Read the model definition and answer for the solid it produces. Units are mm, in the model's axes. A direction names the side the tool comes from. Give positions to 0.01 mm unless a question says otherwise; leave off trailing zeros. Loops run counter-clockwise (first coordinate to the right, second up) from the corner with the lowest first, then second, coordinate; pieces in that order, holes last. Notation, with made-up numbers: (1, -19) - (7, -19) arc R31 cw to (7, 9) - close; hole circle Ø8 at (2.25, 47.25). An arc over 180 degrees is marked (long way). Use a Markdown table: item, result. Add a question column.
Item 1: Consider probe 1 along X at (y, z) = (2.3, 75); probe 2 along Z at (x, y) = (-39, 2.5); probe 3 along X at (y, z) = (-2.5, 42). Determine where each line is inside the solid, lowest interval first. Write a range as [from, to].
Item 2: For a pull along X with two mould halves and no side action, classify faces 1 (the face through (45, 0, 120)), 2 (the face through (50, 0, 59)), 3 (the face through (-1, 0, 70)) as +X half, -X half, draft (parallel to the pull), parting line (faces both ways), or undercut.
Item 3: A cutting plane is placed at C-C (y = -0.85). Determine the outline of the cut face in (x, z), plus the area to 3 significant figures.
Item 4: Which of the six approach directions +Z, -Z, +X, -X, +Y, -Y give full straight-line access (tool end or side, diameter ignored) to faces 4 (the face through (-1, 0, 0)), 5 (the face through (-40, 0, 100)), 6 (the face through (-45, 0, 120)), 7 (the face through (40, 0, 40)), 8 (the face through (45, 1, 75))?
Item 5: Each of these flat-tipped pins is pushed along its axis until it touches: P1, Ø1.8, axis at x = -1.5, y = -1.5, coming from the +Z side; P2, Ø4, axis at x = 44.5, z = 75, coming from the +Y side. Where does it stop, or does it pass through?
Item 6: A cutting plane is placed at B-B (z = 62.5). Determine the outline of the cut face in (x, y), plus the area to 3 significant figures.
Item 7: A cutting plane is placed at A-A (x = -24). Determine the outline of the cut face in (y, z), plus the area to 3 significant figures.
Item 8: A cutting plane is placed at D-D (x = -45). Determine the outline of the cut face in (y, z).
from build123d import *

# Parameters (mm, degrees)
SKETCH1_W           = 80
SKETCH1_H           = 60
BOSS_EXTRUDE1_DEPTH = 3
SKETCH2_R           = 4
CUT_EXTRUDE1_DEPTH  = 2


with BuildPart() as part:
    # Sketch1 → Boss-Extrude1 (new, symmetric)
    with BuildSketch(Plane(origin=(0, 0, 0), x_dir=(1, 0, 0), z_dir=(0, 1, 0))):
        Polygon((-50, 0), (50, 0), (50, -120), (40, -120), (40, -80), (-40, -80), (-40, -120), (-50, -120), align=None)
        with Locations((0, -40)):
            Rectangle(SKETCH1_W, SKETCH1_H, mode=Mode.SUBTRACT)
    extrude(amount=BOSS_EXTRUDE1_DEPTH, both=True)

    # Sketch2 → Cut-Extrude1 (cut)
    with BuildSketch(Plane(origin=(0, 3, 0), x_dir=(1, 0, 0), z_dir=(0, 1, 0))):
        with Locations(Location((-45, -75, 0), (0, 0, 270))):
            Circle(SKETCH2_R)
        with Locations(Location((45, -75, 0), (0, 0, 270))):
            Circle(SKETCH2_R)
    extrude(amount=-CUT_EXTRUDE1_DEPTH, mode=Mode.SUBTRACT)


solid = part.part
Geometry says:
| question | item | result |
|---|---|---|
| 1 | probe 1 | [-50, -49], [-41, 41], [49, 50] |
| 1 | probe 2 | [0, 10], [70, 80] |
| 1 | probe 3 | [-50, -40], [40, 50] |
| 2 | face 1 | draft |
| 2 | face 2 | +X half |
| 2 | face 3 | undercut |
| 3 | outline | (-50, 0) - (50, 0) - (50, 120) - (40, 120) - (40, 80) - (-40, 80) - (-40, 120) - (-50, 120) - close; hole (-40, 10) - (40, 10) - (40, 70) - (-40, 70) - close |
| 3 | area | 4,000 mm² |
| 4 | face 4 | -Z, +X, -X, +Y, -Y |
| 4 | face 5 | +Z, +Y, -Y |
| 4 | face 6 | +Z, +X, -X, +Y, -Y |
| 4 | face 7 | +Y, -Y |
| 4 | face 8 | +Y |
| 5 | P1 | z = 80 |
| 5 | P2 | y = 1 |
| 6 | outline | (-50, -3) - (-40, -3) - (-40, 3) - (-50, 3) - close; (40, -3) - (50, -3) - (50, 3) - (40, 3) - close |
| 6 | area | 120 mm² |
| 7 | outline | (-3, 0) - (3, 0) - (3, 10) - (-3, 10) - close; (-3, 70) - (3, 70) - (3, 80) - (-3, 80) - close |
| 7 | area | 120 mm² |
| 8 | outline | (-3, 0) - (3, 0) - (3, 71) - (1, 71) - (1, 79) - (3, 79) - (3, 120) - (-3, 120) - close |
